```python
from build123d import *

# Parameters (mm, degrees)
BOSS_EXTRUDE1_DEPTH = 20
CUT_EXTRUDE1_DEPTH  = 93.39919136


with BuildPart() as part:
    # Sketch2 → Boss-Extrude1 (new body)
    with BuildSketch(Plane.XY):
        Polygon((90, 0), (90, 15.464828415), (0, 0), (0, -6.378436315), (90, -6.378436315), align=None)
    extrude(amount=BOSS_EXTRUDE1_DEPTH)

    # Sketch5 → Cut-Extrude1 (cut, through all)
    with BuildSketch(Plane(origin=(90, 15.464828415, 0), x_dir=(0, 0, -1), z_dir=(0.985556059, 0.169349504, 0))):
        with BuildLine():
            Line((-15.381941787, 0), (-4.618058213, 0))
            ThreePointArc((-4.618058213, 0), (-10, -4.366552781), (-15.381941787, 0))
        make_face()
    extrude(amount=-CUT_EXTRUDE1_DEPTH, mode=Mode.SUBTRACT)


solid = part.part
```
Input: part model. Units: mm. Frame: model coordinates. Coordinates: 2 decimals unless noted, no trailing zeros. Write each loop counter-clockwise with the first axis right and the second up, starting at its lowest first coordinate (ties: lowest second). Pieces come first, ordered by that corner, then holes.
1) Material intervals for line 1 along Z through (x, y) = (84, 10.5); line 2 along Z through (x, y) = (49.5, 7.75); line 3 along Y through (x, z) = (62.5, 11), sorted ascending.
2) Section A-A on z = 17.25. Output: boundary loops of the cut face in (x, y), and give its area (3 significant figures).
3) Mould query, pull axis Z, two halves, no side actions, for faces 1 (the flat face through (54, 2, 0)), 2 (the flat face through (45.63, 7.84, 2.28)), 3 (the cylindrical face through (45.937, 3.464, 9.895)). Classes: pulls with the +Z half, pulls with the -Z half, needs draft (parallel to the pull), parting line crosses it, or undercut.
4) Section B-B on z = 6.25. Output: boundary loops of the cut face in (x, y), and give its area (3 significant figures).
5) Pin query (flat end, axial travel): pin 1 Ø4 at (x, y) = (9, 4.5) entering from -Z. Return the tip coordinate at first contact, or that it passes through.
Check result:
1. line 1: z = 0 to 7.73, 12.27 to 20
1. line 2: z = 0 to 4.83, 15.17 to 20
1. line 3: y = -6.38 to 6.4
2. outline: (0, -6.38) - (90, -6.38) - (90, 15.46) - (0, 0) - close
2. area: 1,270 mm2
3. face 1: pulls with the -Z half
3. face 2: needs draft
3. face 3: undercut
4. outline: (0, -6.38) - (90, -6.38) - (90, 12.53) - (0, -2.93) - close
4. area: 1,010 mm2
5. pin 1: passes through
